Source: CAD feature listing. Evaluate the final solid. Frame: model axes, mm. Face numbers are marked on the shaded views. A direction names the side the tool comes from. Round coordinates to 2 decimals unless told otherwise and drop trailing zeros. Loops run counter-clockwise (first coordinate to the right, second up) from the corner with the lowest first, then second, coordinate; pieces in that order, holes last. Notation, with made-up numbers: M 87,-28.5 L 126,-28.5 A34 ccw 126,9.5 Z; hole C -12,28 d5. An arc over 180 degrees is marked long. Write each question's results on one line, items separated by ' | '. Start each with the question number.
1. Section B-B on x = 27. Output: boundary loops of the cut face in (y, z) (3 decimals).
2. Ray query, line 1 (X direction, y = 1.25, z = 0); line 2 (X direction, y = -1.75, z = 23.5); line 3 (Y direction, x = 1, z = 3) (3 decimals). Return the intervals inside material, ascending.
3. Section C-C on y = -1.75. Output: boundary loops of the cut face in (x, z).
4. Set-up query: the marked faces 1 and 2. Return all of +Z, -Z, +X, -X, +Y, -Y with unobstructed straight access to the full face (end or side cutting, diameter ignored); none if empty.
5. Contact query for flat-ended pins moving along their axis: pin 1 Ø1 at (x, z) = (49.5, -14.5) entering from -Y; pin 2 Ø1.9 at (x, z) = (10.525, -22.225) entering from +Y; pin 3 Ø1 at (y, z) = (-1.5, 15.5) entering from +X. Output: stop coordinate, or through.
6. Section A-A on z = 0. Give the number of separate pieces and of enclosed holes in the cut face, and give its area (3 significant figures).
from build123d import *

# Parameters (mm, degrees)
SKETCH3_R           = 1.5875
SKETCH3_R_2         = 15.24
BOSS_EXTRUDE1_DEPTH = 3.175
SKETCH4_W           = 63.5
SKETCH4_H           = 6.35
BOSS_EXTRUDE2_DEPTH = 6.35
FILLET1_R           = 3.175


with BuildPart() as part:
    # Sketch3 → Boss-Extrude1 (new body)
    with BuildSketch(Plane(origin=(0, 0, 0), x_dir=(1, 0, 0), z_dir=(0, 1, 0))):
        Polygon((0, 31.75), (0, -31.75), (50.8, -31.75), (58.15, -6.35), (58.15, 6.35), (50.8, 31.75), align=None)
        with Locations(Location((51.8, 0, 0), (0, 0, 270))):
            Circle(SKETCH3_R, mode=Mode.SUBTRACT)
        with Locations(Location((10.525, 22.225, 0), (0, 0, 270))):
            Circle(SKETCH3_R, mode=Mode.SUBTRACT)
        with Locations(Location((10.525, -22.225, 0), (0, 0, 270))):
            Circle(SKETCH3_R, mode=Mode.SUBTRACT)
        with Locations(Location((31.1625, 0, 0), (0, 0, 270))):
            Circle(SKETCH3_R_2, mode=Mode.SUBTRACT)
    extrude(amount=BOSS_EXTRUDE1_DEPTH)

    # Sketch4 → Boss-Extrude2 (add)
    with BuildSketch(Plane.ZY):
        Rectangle(SKETCH4_W, SKETCH4_H)
    extrude(amount=BOSS_EXTRUDE2_DEPTH)

    # Fillet1
    fillet1_edges = [part.edges().sort_by_distance(p)[0] for p in [
        (10.525, 3.175, -23.8125),
        (10.525, 3.175, 20.6375),
        (51.8, 3.175, -1.5875),
    ]]
    fillet(fillet1_edges, radius=FILLET1_R - 0.0001)  # a hair under: the kernel refuses the full size


solid = part.part
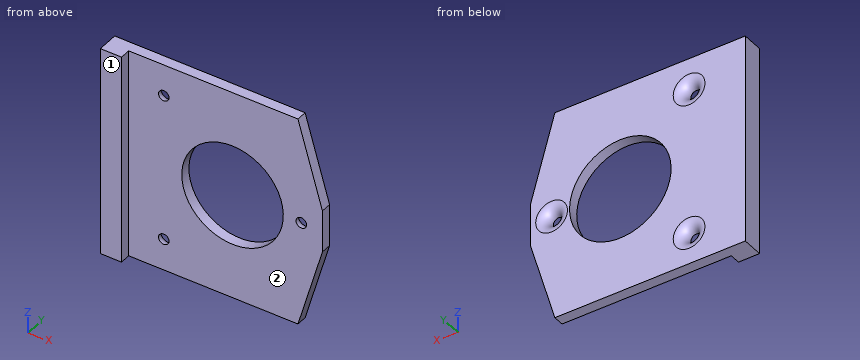
Taken from the geometry:
1) outline: M 0,-31.75 L 3.175,-31.75 L 3.175,-14.661 L 0,-14.661 Z; M 0,14.661 L 3.175,14.661 L 3.175,31.75 L 0,31.75 Z
2) line 1: -6.35 to 15.92, 46.4 to 49.96, 53.64 to 58.15 | line 2: -6.35 to 0 | line 3: 0 to 3.175
3) outline: M -6.35,-31.75 L 0,-31.75 L 0,31.75 L -6.35,31.75 Z
4) face 1: +Z, -Z, +X, -X, -Y | face 2: +Z, -Z, +X, -Y
5) pin 1: y = 0 | pin 2: through | pin 3: x = 0
6) separate pieces: 3 | enclosed holes: 0 | area: 114 mm^2
